Study the drawing (mm; zero at the part's minimum x, y, z) and answer. A direction names the side the tool comes from. Coordinates: 2 decimals unless noted, no trailing zeros. Order: outer loops, then holes, each group sorted by start corner. A loop starts at its lowest first (then second) coordinate and runs counter-clockwise, first axis right, second up.
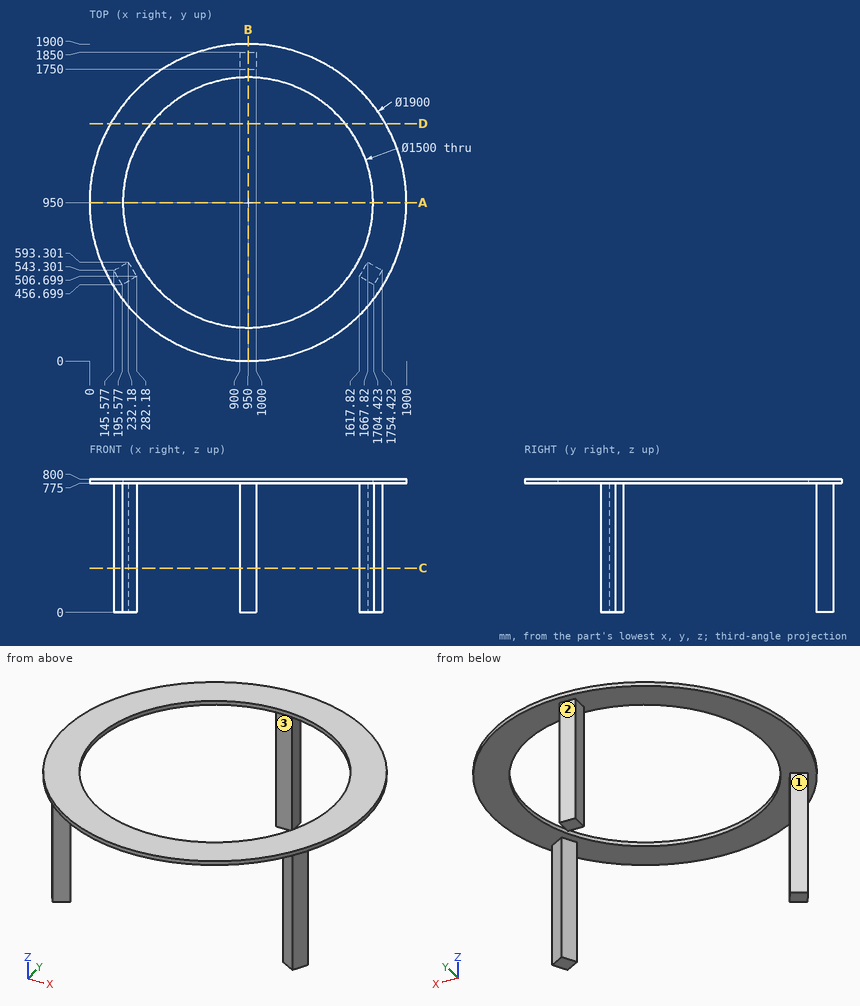
(1) Find section D-D on y = 1422.5. Determine the outline of the cut face in (x, z), then the cut area to 3 significant figures.
(2) Find section A-A on y = 950. Determine the outline of the cut face in (x, z).
(3) A tool of negligible diameter and unlimited length cuts with its end or side. For the marked faces 1, 2 and 3, from which of +Z, -Z, +X, -X, +Y, -Y can it reach the whole face along a straight path? Write none if from no direction.
(4) Find section C-C on z = 266.5. Determine the outline of the cut face in (x, y), then the cut area to 3 significant figures.
(5) Find section B-B on x = 950. Determine the outline of the cut face in (y, z), then the cut area to 3 significant figures.
(6) Given pin 1 Ø6 at (x, z) = (1698, 583) entering from +Y; pin 2 Ø4 at (x, z) = (951, 460.5) entering from -Y; pin 3 Ø3 at (x, y) = (1565.5, 1640) entering from -Z, each flat-ended and moving along its own axis, determine where each tip first touches the part or whether it passes through.
(7) Find the intervals of material crossed by probe 1 along Y at (x, z) = (950, 794); probe 2 along Z at (x, y) = (884.5, 190.5); probe 3 along Y at (x, z) = (990, 347), in increasing order.
Resolved:
1. outline: (125.84, 775) - (367.55, 775) - (367.55, 800) - (125.84, 800) - close; (1532.45, 775) - (1774.16, 775) - (1774.16, 800) - (1532.45, 800) - close
1. area: 12,100 mm2
2. outline: (0, 775) - (200, 775) - (200, 800) - (0, 800) - close; (1700, 775) - (1900, 775) - (1900, 800) - (1700, 800) - close
3. face 1: -Z, -X, +Y
3. face 2: -Z, +X, -X, +Y
3. face 3: -Z, +X, -X, -Y
4. outline: (145.58, 543.3) - (195.58, 456.7) - (282.18, 506.7) - (232.18, 593.3) - close; (900, 1750) - (1000, 1750) - (1000, 1850) - (900, 1850) - close; (1617.82, 506.7) - (1704.42, 456.7) - (1754.42, 543.3) - (1667.82, 593.3) - close
4. area: 30,000 mm2
5. outline: (0, 775) - (200, 775) - (200, 800) - (0, 800) - close; (1700, 775) - (1750, 775) - (1750, 0) - (1850, 0) - (1850, 775) - (1900, 775) - (1900, 800) - (1700, 800) - close
5. area: 87,500 mm2
6. pin 1: stops at y = 577.61
6. pin 2: stops at y = 1750
6. pin 3: stops at z = 775
7. probe 1: y = 0 to 200, 1700 to 1900
7. probe 2: z = 775 to 800
7. probe 3: y = 1750 to 1850
